Autodesk Inventor part; units mm, degrees
ref_plane "YZ Plane" through (0, 0, 0) normal (1, 0, 0) x (0, 1, 0)
ref_plane "XZ Plane" through (0, 0, 0) normal (0, 1, 0) x (-1, 0, 0)
ref_plane "XY Plane" through (0, 0, 0) normal (0, 0, 1) x (1, 0, 0)
sketch "スケッチ1" plane through (0, 0, 0) normal (0, 1, 0) x (-1, 0, 0)
  point P0 (0, 0)
sketch "スケッチ2" plane through (0, 0, 0) normal (0, 1, 0) x (-1, 0, 0)
  line L0 (0.845, -60.969) -> (0.845, -330.969)
  line L1 (0, 0) -> (0, -1.5537)
  line L2 (-202.155, -60.969) -> (-202.155, -330.969)
  arc A0 (-202.155, -330.969) -> (0.845, -330.969) centre (-100.655, -330.969) ccw
  line L3 (0.845, -60.969) -> (0.845, 309.031)
  line L4 (-202.155, -60.969) -> (-202.155, 309.031)
  arc A1 (0.845, 309.031) -> (-202.155, 309.031) centre (-100.655, 309.031) ccw
  dimension "d0" = 270
  dimension "d1" = 203
extrude "押し出し1" add sketch "スケッチ2" against normal blind 10
sketch "スケッチ4" plane through (0, -10, 0) normal (0, -1, 0) x (1, 0, 0)
  line L0 (73.655, -234.969) -> (127.655, -234.969)
  line L1 (127.655, -234.969) -> (127.655, -310.969)
  line L2 (127.655, -310.969) -> (73.655, -310.969)
  line L3 (73.655, -310.969) -> (73.655, -234.969)
  line L4 (202.155, -330.969) -> (202.155, 309.031)
  line L5 (-0.845, 309.031) -> (-0.845, -330.969)
  arc A0 (-0.845, -330.969) -> (202.155, -330.969) centre (100.655, -330.969) ccw
  line L6 (-0.845, -10.969) -> (202.155, -10.969)
  arc A1 (202.155, 309.031) -> (-0.845, 309.031) centre (100.655, 309.031) ccw
  line L7 (73.655, 213.031) -> (127.655, 213.031)
  line L8 (127.655, 213.031) -> (127.655, 289.031)
  line L9 (127.655, 289.031) -> (73.655, 289.031)
  line L10 (73.655, 289.031) -> (73.655, 213.031)
  circle A2 centre (79.655, -299.219) radius 2.75
  line L11 (100.655, -256.1001) -> (100.655, -272.969)
  circle A3 centre (79.655, -245.219) radius 2.75
  circle A4 centre (121.655, -299.219) radius 2.75
  circle A5 centre (121.655, -245.219) radius 2.75
  line L12 (73.655, 213.031) -> (127.655, 213.031)
  line L13 (127.655, 213.031) -> (127.655, 289.031)
  line L14 (127.655, 289.031) -> (73.655, 289.031)
  line L15 (73.655, 289.031) -> (73.655, 213.031)
  circle A6 centre (79.655, 277.281) radius 2.75
  line L16 (100.655, 234.1622) -> (100.655, 251.031)
  circle A7 centre (79.655, 223.281) radius 2.75
  circle A8 centre (121.655, 223.281) radius 2.75
  circle A9 centre (121.655, 277.281) radius 2.75
  point P0 (0, 0)
  dimension "d4" = 74.5
  dimension "d5" = 74.5
  dimension "d6" = 54
  dimension "d7" = 76
  dimension "d8" = 20
  dimension "d9" = 320
  dimension "d17" = 5.5
  dimension "d18" = 11.75
  dimension "d19" = 6
  dimension "d20" = 27
  dimension "d21" = 5.5
  dimension "d22" = 10.25
  dimension "d23" = 6
hole "穴2" at (79.655, -10, -245.219) at (79.655, -10, -299.219) at (121.655, -10, -299.219) at (121.655, -10, -245.219) direction (0, 1, 0) diameter 5.5 end through all
hole "穴3" at (79.655, -10, 223.281) at (121.655, -10, 223.281) at (121.655, -10, 277.281) at (79.655, -10, 277.281) direction (0, 1, 0) diameter 5.5 end through all
sketch "スケッチ6" plane through (0, 0, 0) normal (0, 1, 0) x (1, 0, 0)
  circle A0 centre (153.655, -269.031) radius 6
  circle A1 centre (153.655, -254.031) radius 6
  line L0 (202.155, 330.969) -> (202.155, -309.031)
  arc A2 (-0.845, -309.031) -> (202.155, -309.031) centre (100.655, -309.031) ccw
  point P0 (0, 0)
  dimension "d40" = 12
  dimension "d41" = 12
  dimension "d42" = 15
  dimension "d43" = 48.5
  dimension "d44" = 48.5
  dimension "d45" = 40
hole "穴4" at (153.655, 0, 254.031) at (153.655, 0, 269.031) direction (0, -1, 0) diameter 4.917 end through all
sketch "スケッチ7" plane through (0, 0, 0) normal (0, 1, 0) x (1, 0, 0)
  circle A0 centre (47.655, 290.969) radius 6
  circle A1 centre (47.655, 275.969) radius 6
  arc A2 (202.155, 330.969) -> (-0.845, 330.969) centre (100.655, 330.969) ccw
  line L0 (-0.845, -309.031) -> (-0.845, 330.969)
  point P0 (0, 0)
  dimension "d53" = 12
  dimension "d54" = 12
  dimension "d55" = 15
  dimension "d56" = 40
  dimension "d57" = 48.5
  dimension "d58" = 48.5
hole "穴5" at (47.655, 0, -290.969) at (47.655, 0, -275.969) direction (0, -1, 0) diameter 4.917 end through all
properties part number "sfp_smartboard_lower_deck" material "合板、仕上げ"
Can you work these out from the model? Positions are in its coordinate system, mm. Round coordinates to 2 decimals unless told otherwise and drop trailing zeros. Write each loop counter-clockwise with the first axis right and the second up, starting at its lowest first coordinate (ties: lowest second). Pieces come first, ordered by that corner, then holes. Notation, with made-up numbers: (-4.5, 88.25) -> (50.5, 88.25) arc R11 cw to (50.5, 94.25) -> close; hole circle Ø1 at (75.5, 6). An arc over 180 degrees is marked (long way). One line per question, with ' | ' between items. Start each with the question number.
1) I'm going to push flat-ended pins straight in: P1, Ø6.5, axis at x = 121.655, z = 223.281, coming from the +Y side; P2, Ø4, axis at x = 64, y = -7.5, coming from the +Z side; P3, Ø1, axis at x = 26, y = -7.5, coming from the +Z side. Where does each tip first touch, or does it pass through?
2) I need wall thicknesses on line 1 (X direction, y = -2.5, z = 223) (3 decimals); line 2 (Z direction, x = 123.5, y = -8); line 3 (Z direction, x = 74, y = -3.25). Which ranges of each line are inside material? Lowest first, please. Write a range as [from, to].
3) Suppose I cut it at B-B on x = 26. Write out the boundary of the cut face in (y, z).
4) Suppose I cut it at A-A on y = -1.75. Count the separate pieces of the cut face and the enclosed holes in it, then the cut area to 3 significant figures.
5) Suppose I cut it at C-C on x = 57.5. Write out the boundary of the cut face in (y, z).
Return value:
1) P1: stops at y = 0 | P2: stops at z = 404.43 | P3: stops at z = 378.34
2) line 1: x = [-0.845, 76.919], [82.391, 118.919], [124.391, 202.155] | line 2: z = [-429.86, -301.26], [-297.18, -247.26], [-243.18, 221.24], [225.32, 275.24], [279.32, 407.93] | line 3: z = [-428.91, 406.97]
3) outline: (-10, -399.74) -> (0, -399.74) -> (0, 377.8) -> (-10, 377.8) -> close
4) separate pieces: 1 | enclosed holes: 12 | area: 162,000 mm2
5) outline: (-10, -422.84) -> (0, -422.84) -> (0, 400.9) -> (-10, 400.9) -> close
